```python
from build123d import *

# Parameters (mm, degrees)
ALUMINUM_PLATE_DEPTH         = 3.175
SKETCH5_W                    = 7.394678559
SKETCH5_H                    = 13.40037918
SKETCH5_H_2                  = 13.400379181
CUT_EXTRUDE18_DEPTH          = 3.175
LPATTERN1_COUNT              = 2
LPATTERN1_PITCH              = 70
LPATTERN1_COUNT_DIR2         = 2
LPATTERN1_PITCH_DIR2         = 35.16147
CIRPATTERN1_COUNT            = 4
F_3_0_3_DIAMETER_HOLE5_D     = 3
F_3_0_3_DIAMETER_HOLE5_DEPTH = 25.4
F_3_0_3_DIAMETER_HOLE5_TIP   = 0.901290929
FILLET1_R                    = 1


with BuildPart() as part:
    # Sketch2 → Aluminum plate (new body)
    with BuildSketch(Plane(origin=(0, 0, 0), x_dir=(1, 0, 0), z_dir=(0, 1, 0))):
        with BuildLine():
            Line((58.411953225, -27.670918752), (-21.588046771, -27.670918749))
            ThreePointArc((-21.588046771, -27.670918749), (-25.123580677, -26.206452654), (-26.588046771, -22.670918748))
            Line((-26.588046771, -22.670918748), (-26.588046767, 57.329032922))
            ThreePointArc((-26.588046767, 57.329032922), (-25.123563586, 60.864583915), (-21.587998438, 62.329032922))
            Line((-21.587998438, 62.329032922), (58.412001558, 62.328259655))
            ThreePointArc((58.412001558, 62.328259655), (61.947504222, 60.863776475), (63.411953229, 57.328259655))
            Line((63.411953229, 57.328259655), (63.411953225, -22.670918752))
            ThreePointArc((63.411953225, -22.670918752), (61.947487131, -26.206452658), (58.411953225, -27.670918752))
        make_face()
        Polygon((39.839453224, -4.0986466), (-3.015546772, -4.098646598), (-3.01554677, 38.756353402), (39.83945323, 38.7563534), align=None, mode=Mode.SUBTRACT)
    extrude(amount=ALUMINUM_PLATE_DEPTH)

    # Sketch5 → Cut-Extrude18 (cut)
    with BuildSketch(Plane(origin=(0, 3.175, 0), x_dir=(1, 0, 0), z_dir=(0, 1, 0))):
        with Locations((43.53679251, 2.60154299)):
            Rectangle(SKETCH5_W, SKETCH5_H)
        with Locations((43.53679251, 32.056163809)):
            Rectangle(SKETCH5_W, SKETCH5_H_2)
    extrude(amount=-CUT_EXTRUDE18_DEPTH, mode=Mode.SUBTRACT)

    # Sketch12 → 3.0 _3_ Diameter Hole3 (revolve, cut)
    with BuildSketch(Plane(origin=(-16.588046767, 3.175, -34.909587365), x_dir=(0, 0, 1), z_dir=(1, 0, 0))):
        Polygon((0, 0), (0, 26.301290929), (1.5, 25.4), (1.5, 0), align=None)
    f_3_0_3_diameter_hole3 = revolve(axis=Axis((-16.588046767, 9.525, -34.909587365), (0, -1, 0)), mode=Mode.SUBTRACT)

    # LPattern1: 3.0 _3_ Diameter Hole3 2 × 2
    with Locations(*[(i * LPATTERN1_PITCH, 0, j * LPATTERN1_PITCH_DIR2) for i in range(LPATTERN1_COUNT) for j in range(LPATTERN1_COUNT_DIR2) if (i, j) != (0, 0)]):
        add(f_3_0_3_diameter_hole3, mode=Mode.SUBTRACT)

    # Sketch14 → 3.0 _3_ Diameter Hole4 (revolve, cut)
    with BuildSketch(Plane(origin=(42.221953226, 3.175, -17.329161252), x_dir=(0, 0, 1), z_dir=(1, 0, 0))):
        Polygon((0, 0), (0, 26.301290929), (1.5, 25.4), (1.5, 0), align=None)
    f_3_0_3_diameter_hole4 = revolve(axis=Axis((42.221953226, 9.525, -17.329161252), (0, -1, 0)), mode=Mode.SUBTRACT)

    # CirPattern1: 3.0 _3_ Diameter Hole4 ×4 about axis
    cirpattern1_axis = Axis((18.411953227, 0, -17.328853403), (0, 1, 0))
    for i in range(1, CIRPATTERN1_COUNT):
        add(f_3_0_3_diameter_hole4.rotate(cirpattern1_axis, i * 360 / CIRPATTERN1_COUNT), mode=Mode.SUBTRACT)

    # 3.0 _3_ Diameter Hole5
    with Locations(Plane.XZ):
        with Locations((-19.688046767, -54.730581251), (56.511953233, -54.730581251), (56.511953233, 20.072418749), (-19.688046767, 20.072418749)):
            Hole(F_3_0_3_DIAMETER_HOLE5_D / 2, depth=F_3_0_3_DIAMETER_HOLE5_DEPTH)
            with Locations((0, 0, -(F_3_0_3_DIAMETER_HOLE5_DEPTH + F_3_0_3_DIAMETER_HOLE5_TIP / 2))):  # 118° drill point
                Cone(0, F_3_0_3_DIAMETER_HOLE5_D / 2, F_3_0_3_DIAMETER_HOLE5_TIP, mode=Mode.SUBTRACT)

    # Fillet1
    fillet1_edges = [part.edges().sort_by_distance(p)[0] for p in [
        (-25.123563586, 3.175, -60.864583915),
        (18.41200156, 0, -62.328646289),
        (61.947504222, 0, -60.863776475),
        (-26.588046769, 3.175, -17.329057087),
        (-25.123580677, 3.175, 26.206452654),
        (18.411953227, 3.175, 27.67091875),
        (61.947487131, 3.175, 26.206452658),
        (63.411953227, 3.175, -17.328670452),
        (61.947504222, 3.175, -60.863776475),
        (18.41200156, 3.175, -62.328646289),
        (63.411953227, 0, -17.328670452),
        (61.947487131, 0, 26.206452658),
        (18.411953227, 0, 27.67091875),
        (-25.123580677, 0, 26.206452654),
        (-26.588046769, 0, -17.329057087),
        (-25.123563586, 0, -60.864583915),
    ]]
    fillet(fillet1_edges, radius=FILLET1_R)


solid = part.part
```
Here's how the part is built. I have some questions about the finished solid (model axes, mm). A direction names the side the tool comes from. Coordinates: 2 decimals unless noted, no trailing zeros. Loops run counter-clockwise (first coordinate to the right, second up) from the corner with the lowest first, then second, coordinate; pieces in that order, holes last. Notation, with made-up numbers: (30.5, 72.5) - (87.5, 72.5) arc R19 cw to (87.5, 88.5) - close; hole circle Ø2 at (36.25, -3.75). An arc over 180 degrees is marked (long way). Return JSON: item names as keys, results as strings. Group by question number.
Item 1: Will this pin go through, and if not, where does the flat tip stop? P1, Ø4, axis at x = 42.22, z = -17.33, coming from the +Y side (3 decimals).
Item 2: On a 3-axis mill with a long thin cutter (end or side, diameter ignored), from which of +Z, -Z, +X, -X, +Y, -Y can I reach the whole of each face in a straight line? I mean faces 4 (the face through (43, 2, -9.302)), 5 (the face through (61.986, 1.579, 26.167)). Say none if no direction works.
Item 3: I need wall thicknesses on line 1 (Z direction, x = 40, y = 2.05); line 2 (Z direction, x = 41.5, y = 3.05); line 3 (X direction, y = 1.35, z = 1). Which ranges of each line are inside material? Lowest first, please. Write a range as from..to.
Item 4: If we section it at A-A on z = -27.5: Write out the boundary of the cut face in (x, y) (3 decimals).
Item 5: We'd pull the mould along X, two halves only. Please class faces 1 (the face through (61.91, 1.58, -60.9)), 2 (the face through (18.22, 1.61, -39.65)), 3 (the face through (-25.16, 1.58, -60.83)): +X half, -X half, draft (parallel to the pull), parting line (faces both ways), or undercut.
Calculated:
{
 "1": {"P1": "stops at y = 3.175"},
 "2": {"face 4": "+Y, -Y", "face 5": "+Z, +X, +Y, -Y"},
 "3": {"line 1": "z = -62.33..-38.76, -25.36..-9.3, 4.1..27.67", "line 2": "z = -61.81..-38.76, -25.36..-18.64, -16.01..-9.3, 4.1..27.16", "line 3": "x = -26.59..-17.89, -15.29..-3.02, 47.23..52.11, 54.71..63.41"},
 "4": {"outline": "(-26.588, 1) arc R1 ccw to (-25.588, 0) - (-3.016, 0) - (-3.016, 3.175) - (-25.588, 3.175) arc R1 ccw to (-26.588, 2.175) - close; (47.234, 0) - (62.412, 0) arc R1 ccw to (63.412, 1) - (63.412, 2.175) arc R1 ccw to (62.412, 3.175) - (47.234, 3.175) - close"},
 "5": {"face 1": "+X half", "face 2": "undercut", "face 3": "-X half"}
}
